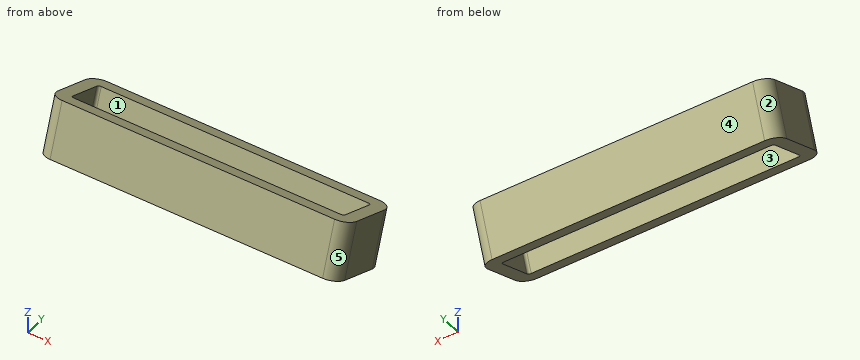
from build123d import *

# Parameters (mm, degrees)
PAD004_DEPTH    = 11.25
POCKET001_DEPTH = 5
FILLET002_R     = 1


with BuildPart() as part:
    # Sketch033 → Pad004 (new body, symmetric)
    with BuildSketch(Plane.YZ):
        Polygon((27.3746847171, -17.3800460051), (32.2053280153, -19.0155536712), (30.9225769046, -22.8042935129), (26.0919336064, -21.1687858467), align=None)
    extrude(amount=PAD004_DEPTH, both=True)

    # Sketch034 (on Face1 of Pad004) → Pocket001 (cut)
    with BuildSketch(Plane(origin=(0, -2.463969707, -7.2775927611), x_dir=(0, -0.9471849604, 0.3206877777), z_dir=(0, 0.3206877777, 0.9471849604))):
        with BuildLine():
            Line((-35.4024579896, 10.25), (-32.7024579896, 10.25))
            ThreePointArc((-32.5024579896, 10.05), (-32.5610366334, 10.1914213562), (-32.7024579896, 10.25))
            Line((-32.5024579896, 10.05), (-32.5024579896, -10.05))
            ThreePointArc((-32.7024579896, -10.25), (-32.5610366334, -10.1914213562), (-32.5024579896, -10.05))
            Line((-32.7024579896, -10.25), (-35.4024579896, -10.25))
            ThreePointArc((-35.6024579896, -10.05), (-35.5438793458, -10.1914213562), (-35.4024579896, -10.25))
            Line((-35.6024579896, -10.05), (-35.6024579896, 10.05))
            ThreePointArc((-35.4024579896, 10.25), (-35.5438793458, 10.1914213562), (-35.6024579896, 10.05))
        make_face()
    extrude(amount=-POCKET001_DEPTH, mode=Mode.SUBTRACT)

    # Fillet002
    fillet002_edges = [part.edges().sort_by_distance(p)[0] for p in [
        (11.25, 31.563952, -20.909924),
        (11.25, 26.733309, -19.274416),
        (-11.25, 31.563952, -20.909924),
        (-11.25, 26.733309, -19.274416),
    ]]
    fillet(fillet002_edges, radius=FILLET002_R)


solid = part.part
Source: CAD feature listing. Evaluate the final solid. Frame: model axes, mm. Face numbers are marked on the shaded views. A direction names the side the tool comes from. Give positions to 0.01 mm unless a question says otherwise; leave off trailing zeros. Order: outer loops, then holes, each group sorted by start corner. A loop starts at its lowest first (then second) coordinate and runs counter-clockwise, first axis right, second up. Notation, with made-up numbers: (24, -1.75) -> (47, -1.75) arc R10 ccw to (47, 13.25) -> close; hole circle Ø11 at (16.5, 54.5). An arc over 180 degrees is marked (long way). Write item = value, one per line.
Q1. Set-up query: the marked faces 1 and 2. Return all of +Z, -Z, +X, -X, +Y, -Y with unobstructed straight access to the full face (end or side cutting, diameter ignored); none if empty.
Data:
face_1 = +Z
face_2 = -Z, -X, +Y
Q2. Pull-direction query (X, two-part tool) for the marked faces 3, 4 and 5; classes: released by +X, released by -X, zero draft, split by the parting line, or undercut.
Data:
face_3 = undercut
face_4 = zero draft
face_5 = released by +X
Q3. Cut plane A-A, the plane x = -2. Output: boundary loops of the cut face in (y, z), and give its area (3 significant figures).
Data:
outline = (26.09, -21.17) -> (27.04, -21.49) -> (28.32, -17.7) -> (27.37, -17.38) -> close; (29.98, -22.48) -> (30.92, -22.8) -> (32.21, -19.02) -> (31.26, -18.69) -> close
area = 8.00 mm^2
Q4. Pin query (flat end, axial travel): pin 1 (1 mm diameter, centred on x = 4.5, y = 29, fed in from +Z). Return the tip coordinate at first contact, or that it passes through.
Data:
pin_1 = through
Q5. Material intervals for line 1 (X direction, y = 30.5, z = -19.8); line 2 (Y direction, x = -1.5, z = -20.25); line 3 (Y direction, x = 9.25, z = -20.45), sorted ascending. Write a range as from..to.
Data:
line_1 = -11.25..-10.25, 10.25..11.25
line_2 = 26.4..27.46, 30.73..31.79
line_3 = 26.34..27.39, 30.66..31.72
